Read the model definition and answer for the solid it produces. Units are mm, in the model's axes. Give positions to 0.01 mm unless a question says otherwise; leave off trailing zeros. Write each loop counter-clockwise with the first axis right and the second up, starting at its lowest first coordinate (ties: lowest second). Pieces come first, ordered by that corner, then holes. Notation, with made-up numbers: (72.5, 53.25) -> (106.5, 53.25) arc R30 cw to (106.5, 90.25) -> close; hole circle Ø2 at (8, 34.25). An arc over 180 degrees is marked (long way). Put each result on its own line as item: value. Start each with the question number.
from build123d import *

# Parameters (mm, degrees)
CROQUIS1_W              = 33
CROQUIS1_H              = 18
CROQUIS1_R              = 0.5
SALIENTE_EXTRUIR1_DEPTH = 1


with BuildPart() as part:
    # Croquis1 → Saliente-Extruir1 (new body)
    with BuildSketch(Plane(origin=(0, 0, 0), x_dir=(1, 0, 0), z_dir=(0, 1, 0))):
        with Locations((-7.138495914, 0)):
            Rectangle(CROQUIS1_W, CROQUIS1_H)
        with Locations((-22.638495914, 1)):
            Circle(CROQUIS1_R, mode=Mode.SUBTRACT)
        with Locations((-22.638495914, 3)):
            Circle(CROQUIS1_R, mode=Mode.SUBTRACT)
        with Locations((-22.638495914, 5)):
            Circle(CROQUIS1_R, mode=Mode.SUBTRACT)
        with Locations((-20.638495914, 8)):
            Circle(CROQUIS1_R, mode=Mode.SUBTRACT)
        with Locations((-18.098495914, 8)):
            Circle(CROQUIS1_R, mode=Mode.SUBTRACT)
        with Locations((-15.558495914, 8)):
            Circle(CROQUIS1_R, mode=Mode.SUBTRACT)
        with Locations((-13.018495914, 8)):
            Circle(CROQUIS1_R, mode=Mode.SUBTRACT)
        with Locations((-10.478495914, 8)):
            Circle(CROQUIS1_R, mode=Mode.SUBTRACT)
        with Locations((-7.938495914, 8)):
            Circle(CROQUIS1_R, mode=Mode.SUBTRACT)
        with Locations((-5.398495914, 8)):
            Circle(CROQUIS1_R, mode=Mode.SUBTRACT)
        with Locations((-2.858495914, 8)):
            Circle(CROQUIS1_R, mode=Mode.SUBTRACT)
        with Locations((-0.318495914, 8)):
            Circle(CROQUIS1_R, mode=Mode.SUBTRACT)
        with Locations((2.221504086, 8)):
            Circle(CROQUIS1_R, mode=Mode.SUBTRACT)
        with Locations((4.761504086, 8)):
            Circle(CROQUIS1_R, mode=Mode.SUBTRACT)
        with Locations((7.301504086, 8)):
            Circle(CROQUIS1_R, mode=Mode.SUBTRACT)
        with Locations((7.301504086, -8)):
            Circle(CROQUIS1_R, mode=Mode.SUBTRACT)
        with Locations((4.761504086, -8)):
            Circle(CROQUIS1_R, mode=Mode.SUBTRACT)
        with Locations((2.221504086, -8)):
            Circle(CROQUIS1_R, mode=Mode.SUBTRACT)
        with Locations((-0.318495914, -8)):
            Circle(CROQUIS1_R, mode=Mode.SUBTRACT)
        with Locations((-2.858495914, -8)):
            Circle(CROQUIS1_R, mode=Mode.SUBTRACT)
        with Locations((-5.398495914, -8)):
            Circle(CROQUIS1_R, mode=Mode.SUBTRACT)
        with Locations((-7.938495914, -8)):
            Circle(CROQUIS1_R, mode=Mode.SUBTRACT)
        with Locations((-10.478495914, -8)):
            Circle(CROQUIS1_R, mode=Mode.SUBTRACT)
        with Locations((-13.018495914, -8)):
            Circle(CROQUIS1_R, mode=Mode.SUBTRACT)
        with Locations((-15.558495914, -8)):
            Circle(CROQUIS1_R, mode=Mode.SUBTRACT)
        with Locations((-18.098495914, -8)):
            Circle(CROQUIS1_R, mode=Mode.SUBTRACT)
        with Locations((-20.638495914, -8)):
            Circle(CROQUIS1_R, mode=Mode.SUBTRACT)
        with Locations((-22.638495914, -5)):
            Circle(CROQUIS1_R, mode=Mode.SUBTRACT)
        with Locations((-22.638495914, -3)):
            Circle(CROQUIS1_R, mode=Mode.SUBTRACT)
        with Locations((-22.638495914, -1)):
            Circle(CROQUIS1_R, mode=Mode.SUBTRACT)
    extrude(amount=SALIENTE_EXTRUIR1_DEPTH)


solid = part.part
1) Straight lines are drawn through the part: line 1 (X direction, y = 0.6, z = -3); line 2 (Z direction, x = -2.5, y = 0.85); line 3 (Z direction, x = -5.5, y = 0.9). For each, find the intervals that lie inside material, in ascending order. Write a range as [from, to].
2) A cutting plane is placed at B-B on z = 3. Give the vertices of the cut face in (x, y).
3) For a pull along Z with two mould halves and no side action, classify faces 1 (the face through (-2.967, 0.493, 8.488)), 2 (the face through (-23.638, 0.5, 0.1)) as pulls with the +Z half, pulls with the -Z half, needs draft (parallel to the pull), parting line crosses it, or undercut.
4) A cutting plane is placed at A-A on y = 0.85. State how many separate pieces and enclosed holes the cut face has, and give its area (3 significant figures).
Results found:
1. line 1: x = [-23.64, -23.14], [-22.14, 9.36]
1. line 2: z = [-9, -8.35], [-7.65, 7.65], [8.35, 9]
1. line 3: z = [-9, -8.49], [-7.51, 7.51], [8.49, 9]
2. outline: (-23.64, 0) -> (-23.14, 0) -> (-23.14, 1) -> (-23.64, 1) -> close; (-22.14, 0) -> (9.36, 0) -> (9.36, 1) -> (-22.14, 1) -> close
3. face 1: undercut
3. face 2: needs draft
4. separate pieces: 1
4. enclosed holes: 30
4. area: 570 mm²
